Geometry: see drawing. Coordinates: mm, zero at the bounding-box minimum. A direction names the side the tool comes from. Give positions to 0.01 mm unless a question says otherwise; leave off trailing zeros. Write each loop counter-clockwise with the first axis right and the second up, starting at its lowest first coordinate (ties: lowest second). Pieces come first, ordered by that corner, then holes. Notation, with made-up numbers: (80, 21.5) - (97, 21.5) arc R19 ccw to (97, 57.5) - close; hole circle Ø10 at (52.5, -19). An arc over 180 degrees is marked (long way). Use CSV: the item, a comma, the result in double quotes. Start each with the question number.
(1) First-contact query: pin 1 Ø10 at (x, y) = (128, 98) entering from +Z; pin 2 Ø3 at (y, z) = (86.5, 58) entering from +X; pin 3 Ø15 at (x, z) = (114, 53) entering from -Y. Flat tips, straight axial feed; report the tip coordinate or a pass-through.
(2) Reachability of the marked faces 5, 6, 7 and 8 from +Z, -Z, +X, -X, +Y, -Y: full face, straight path, thin tool, end or side. Return the list, or none.
(3) Section D-D on x = 141. Output: boundary loops of the cut face in (y, z), and give its area (3 significant figures).
(4) Section A-A on x = 120. Output: boundary loops of the cut face in (y, z), and give its area (3 significant figures).
(5) Draft query along Z for the marked faces 1, 2, 3 and 4. Return one class per face: released by +Z, released by -Z, zero draft, split by the parting line, or undercut.
(6) Section C-C on y = 15. Output: boundary loops of the cut face in (x, z).
(7) Line query: probe 1 along Y at (x, z) = (120, 11); probe 2 along Y at (x, z) = (120, 13.5); probe 3 along Z at (x, y) = (13, 79). Output: solid intervals per line, ascending. Write a range as [from, to].
(8) Section B-B on z = 14.5. Output: boundary loops of the cut face in (x, y).
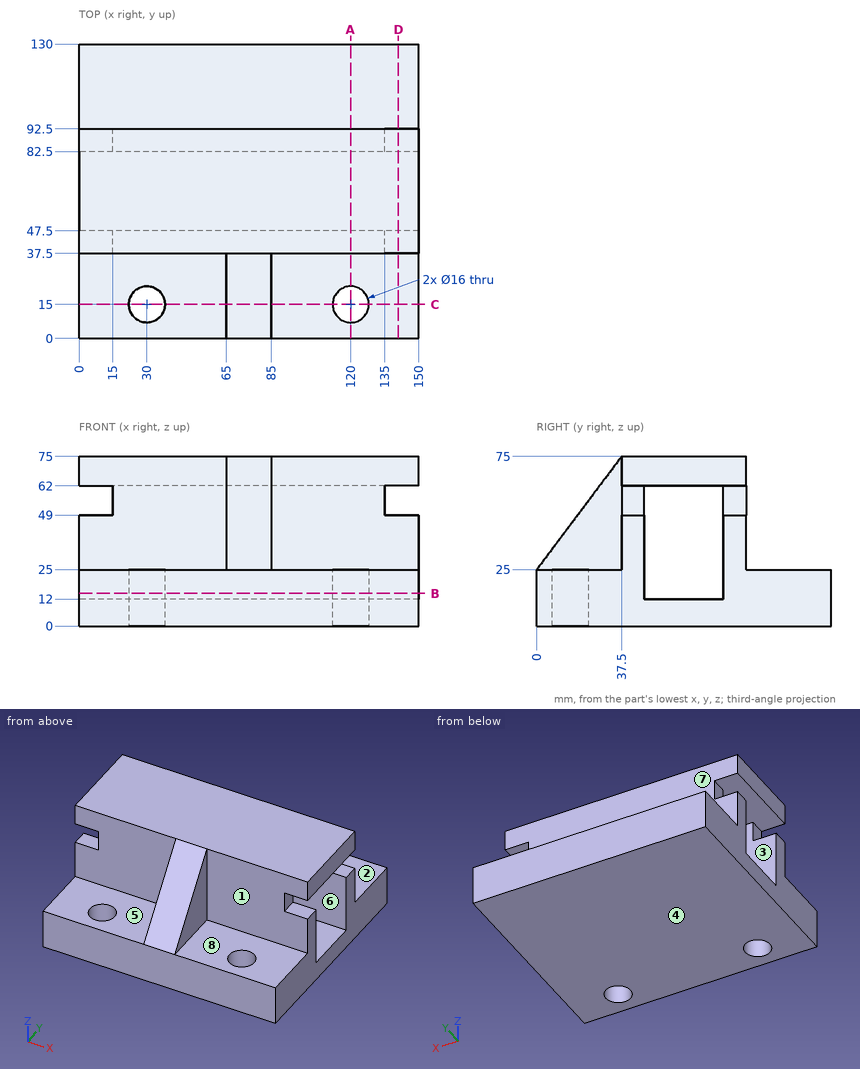
Check values:
1,pin 1,"stops at z = 25"
1,pin 2,"stops at x = 135"
1,pin 3,"stops at y = 37.5"
2,face 5,"+Z, -X, -Y"
2,face 6,"+X, -X"
2,face 7,"+Z, +X, -X, +Y"
2,face 8,"+Z, +X, -Y"
3,outline,"(0, 0) - (130, 0) - (130, 25) - (92.5, 25) - (92.5, 49) - (82.5, 49) - (82.5, 12) - (47.5, 12) - (47.5, 49) - (37.5, 49) - (37.5, 25) - (0, 25) - close; (37.5, 62) - (92.5, 62) - (92.5, 75) - (37.5, 75) - close"
3,area,"3,990 mm²"
4,outline,"(0, 0) - (7, 0) - (7, 25) - (0, 25) - close; (23, 0) - (130, 0) - (130, 25) - (92.5, 25) - (92.5, 75) - (37.5, 75) - (37.5, 25) - (23, 25) - close; hole (47.5, 12) - (82.5, 12) - (82.5, 62) - (47.5, 62) - close"
4,area,"3,850 mm²"
5,face 1,"zero draft"
5,face 2,"released by +Z"
5,face 3,"undercut"
5,face 4,"released by -Z"
6,outline,"(0, 0) - (22, 0) - (22, 25) - (0, 25) - close; (38, 0) - (112, 0) - (112, 25) - (85, 25) - (85, 45) - (65, 45) - (65, 25) - (38, 25) - close; (128, 0) - (150, 0) - (150, 25) - (128, 25) - close"
7,probe 1,"y = [0, 7], [23, 130]"
7,probe 2,"y = [0, 7], [23, 47.5], [82.5, 130]"
7,probe 3,"z = [0, 12], [62, 75]"
8,outline,"(0, 0) - (150, 0) - (150, 47.5) - (0, 47.5) - close; (0, 82.5) - (150, 82.5) - (150, 130) - (0, 130) - close; hole circle Ø16 at (30, 15); hole circle Ø16 at (120, 15)"
